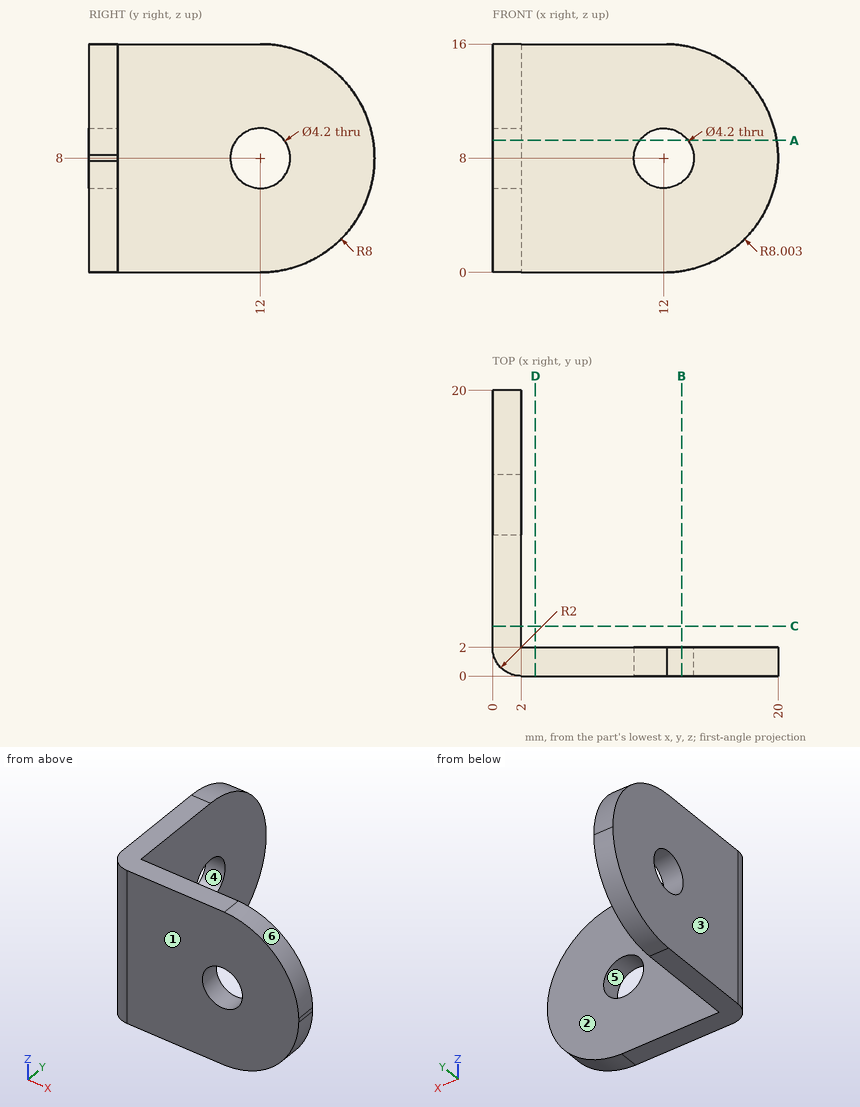
Answer from the drawing. Dimensions are ordinates in mm from the lowest x, y and z of the part. A direction names the side the tool comes from. Round coordinates to 2 decimals unless told otherwise and drop trailing zeros. Loops run counter-clockwise (first coordinate to the right, second up) from the corner with the lowest first, then second, coordinate; pieces in that order, holes last.
Q1. Section A-A on z = 9.25 is taken. Write down the section's boundary in (x, y) (1 decimal).
Q2. Consider probe 1 along Z at (x, y) = (12, 1.55); probe 2 along Y at (x, z) = (8.5, 5.25). Determine where each line is inside the solid, lowest interval first.
Q3. Section B-B on x = 13.25 is taken. Write down the section's boundary in (y, z) (1 decimal).
Q4. Each of these flat-tipped pins is pushed along its axis until it touches: pin 1 (1 mm diameter, centred on y = 13, z = 8.5, fed in from -X); pin 2 (3 mm diameter, centred on x = 11.5, z = 13, fed in from +Y); pin 3 (5 mm diameter, centred on y = 13.5, z = 8, fed in from +X). Where does it stop, or does it pass through?
Q5. Which of the six approach directions +Z, -Z, +X, -X, +Y, -Y give full straight-line access (tool end or side, diameter ignored) to the marked faces 1 and 2?
Q6. Determine the mould class of the marked faces 3, 4, 5 and 6 for opening direction Z: released by +Z, released by -Z, zero draft, split by the parting line, or undercut.
Q7. Section C-C on y = 3.5 is taken. Write down the section's boundary in (x, z).
Output:
1. outline: (0, 2) arc R2 ccw to (2, 0) - (10.3, 0) - (10.3, 2) - (2, 2) - (2, 10.3) - (0, 10.3) - close; (0, 13.7) - (2, 13.7) - (2, 19.9) - (0, 19.9) - close; (13.7, 0) - (19.9, 0) - (19.9, 2) - (13.7, 2) - close
2. probe 1: z = 0 to 5.9, 10.1 to 16
2. probe 2: y = 0 to 2
3. outline: (0, 0.1) - (2, 0.1) - (2, 6.3) - (0, 6.3) - close; (0, 9.7) - (2, 9.7) - (2, 15.9) - (0, 15.9) - close
4. pin 1: passes through
4. pin 2: stops at y = 2
4. pin 3: stops at x = 2
5. face 1: +Z, -Z, +X, -X, -Y
5. face 2: +Z, -Z, +X, +Y
6. face 3: zero draft
6. face 4: undercut
6. face 5: undercut
6. face 6: released by +Z
7. outline: (0, 0) - (2, 0) - (2, 16) - (0, 16) - close
